Could you check a few things on this model? Use its own coordinates, in mm. Face numbers are marked on the shaded views. A direction names the side the tool comes from. Coordinates: 2 decimals unless noted, no trailing zeros. Write each loop counter-clockwise with the first axis right and the second up, starting at its lowest first coordinate (ties: lowest second). Pieces come first, ordered by that corner, then holes.
```python
from build123d import *

# Parameters (mm, degrees)
F1_DEPTH  = 41
F2_R      = 24.4692351537
F2_R_2    = 16.3
F3_DEPTH  = 25
F4_R      = 21.9531203574
F4_R_2    = 15
F5_DEPTH  = 9
F6_R      = 16.3
F7_DEPTH  = 7
F8_R      = 2.85
F9_DEPTH  = 41.001
F10_R     = 13.8
F11_DEPTH = 2.3
F12_R     = 6
F13_DEPTH = 41.001
F14_R     = 6.5
F15_DEPTH = 29
F16_R     = 2.5
F17_DEPTH = 13
F18_R     = 2.5
F19_DEPTH = 14.4
F21_D     = 4.2
F21_DEPTH = 8
F21_TIP   = 1.2618073
F22_R     = 3
F23_DEPTH = 29


with BuildPart() as f1:
    # F0 (on Front) → F1 (new body)
    with BuildSketch(Plane.XZ):
        Polygon((-18, -10.3923048454), (0, -20.7846096908), (18, -10.3923048454), (18, 10.3923048454), (0, 20.7846096908), (-18, 10.3923048454), align=None)
    extrude(amount=-F1_DEPTH)

    # F2 (on face) → F3 (cut)
    with BuildSketch(Plane(origin=(0, 41, 0), x_dir=(-1, 0, 0), z_dir=(0, 1, 0))):
        Circle(F2_R)
        Circle(F2_R_2, mode=Mode.SUBTRACT)
    extrude(amount=-F3_DEPTH, mode=Mode.SUBTRACT)

    # F4 (on face) → F5 (cut)
    with BuildSketch(Plane(origin=(0, 41, 0), x_dir=(-1, 0, 0), z_dir=(0, 1, 0))):
        Circle(F4_R)
        Circle(F4_R_2, mode=Mode.SUBTRACT)
    extrude(amount=-F5_DEPTH, mode=Mode.SUBTRACT)

    # F6 (on face) → F7 (join)
    with BuildSketch(Plane(origin=(0, 41, 0), x_dir=(-1, 0, 0), z_dir=(0, 1, 0))):
        Circle(F6_R)
    extrude(amount=-F7_DEPTH)

    # F8 (on face) → F9 (cut, through all)
    with BuildSketch(Plane.XZ):
        with Locations((8.5, 0)):
            Circle(F8_R)
        with Locations((4.87, -6.95)):
            Circle(F8_R)
    extrude(amount=-F9_DEPTH, mode=Mode.SUBTRACT)

    # F10 (on face) → F11 (cut)
    with BuildSketch(Plane(origin=(0, 41, 0), x_dir=(-1, 0, 0), z_dir=(0, 1, 0))):
        Circle(F10_R)
    extrude(amount=-F11_DEPTH, mode=Mode.SUBTRACT)

    # F12 (on face) → F13 (cut, through all)
    with BuildSketch(Plane.XZ):
        with Locations((-5, 0)):
            Circle(F12_R)
    extrude(amount=-F13_DEPTH, mode=Mode.SUBTRACT)

    # F14 (on face) → F15 (cut)
    with BuildSketch(Plane(origin=(0, 38.7, 0), x_dir=(-1, 0, 0), z_dir=(0, 1, 0))):
        with Locations((5, 0)):
            Circle(F14_R)
    extrude(amount=-F15_DEPTH, mode=Mode.SUBTRACT)

    # F16 (on face) → F17 (cut)
    with BuildSketch(Plane.XZ):
        with Locations((-0.1, 14.8379019182)):
            Circle(F16_R)
    extrude(amount=-F17_DEPTH, mode=Mode.SUBTRACT)

    # F18 (on face) → F19 (cut)
    with BuildSketch(Plane.XZ):
        with Locations((0.1, -14.8379019182)):
            Circle(F18_R)
    extrude(amount=-F19_DEPTH, mode=Mode.SUBTRACT)

    # F21
    with Locations(Plane(origin=(9, 0, 15.5884572681), x_dir=(0.8660254038, 0, -0.5), z_dir=(0.5, 0, 0.8660254038))):
        with Locations((4.4923048454, 5.9)):
            Hole(F21_D / 2, depth=F21_DEPTH)
            with Locations((0, 0, -(F21_DEPTH + F21_TIP / 2))):  # 118° drill point
                Cone(0, F21_D / 2, F21_TIP, mode=Mode.SUBTRACT)

    # F22 (on face) → F23 (cut)
    with BuildSketch(Plane(origin=(0, 38.7, 0), x_dir=(-1, 0, 0), z_dir=(0, 1, 0))):
        with Locations((-4.62, 7.15)):
            Circle(F22_R)
    extrude(amount=-F23_DEPTH, mode=Mode.SUBTRACT)


solid = f1.part
```
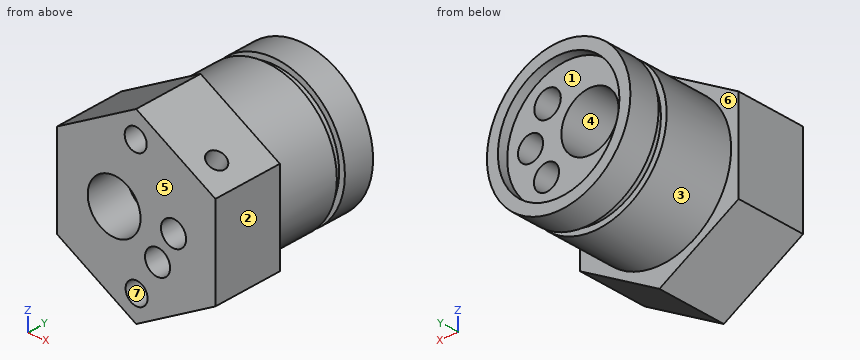
1. Please list where these lines run through material, in increasing order: line 1 along Z through (x, y) = (0, 6); line 2 along Y through (x, z) = (-16, -1.5); line 3 along Y through (x, z) = (0.5, 16).
Verdict:
line 1: z = -20.78 to -17.34, -12.34 to -3.32, 3.32 to 12.34, 17.34 to 20.78
line 2: y = 0 to 32, 34 to 41
line 3: y = 13 to 32, 34 to 41
2. For pin 1 (10 mm diameter, centred on x = -11.5, z = -4, fed in from +Y); pin 2 (17 mm diameter, centred on x = -5, z = 0, fed in from +Y); pin 3 (8 mm diameter, centred on x = -5, y = 22.5, fed in from +Z); pin 4 (8 mm diameter, centred on x = -7.5, y = 22, fed in from -Z), each with a flat end and sliding along its axis, tell me the tip position at first contact or that it passes through.
Verdict:
pin 1: stops at y = 41
pin 2: stops at y = 38.7
pin 3: stops at z = 16.27
pin 4: stops at z = -15.92
3. On a 3-axis mill with a long thin cutter (end or side, diameter ignored), from which of +Z, -Z, +X, -X, +Y, -Y can I reach the whole of each face in a straight line? I mean the marked faces 5, 6 and 7. Say none if no direction works.
Verdict:
face 5: +Z, -Z, +X, -X, -Y
face 6: +Y
face 7: -Y
4. I want a section at C-C on y = 28. Please give me the cut outline in (x, z).
Verdict:
outline: circle Ø32.6 at (0, 0); hole circle Ø13 at (-5, 0); hole circle Ø6 at (4.62, 7.15); hole circle Ø5.7 at (4.87, -6.95); hole circle Ø5.7 at (8.5, 0)
5. I want a section at B-B on x = 4.87. Please give me the cut outline in (y, z).
Verdict:
outline: (0, -17.97) - (16, -17.97) - (16, -15.56) - (32, -15.56) - (32, -14.19) - (34, -14.19) - (34, -15.56) - (41, -15.56) - (41, -12.91) - (38.7, -12.91) - (38.7, -9.8) - (0, -9.8) - close; (0, -4.1) - (38.7, -4.1) - (38.7, 4.16) - (9.7, 4.16) - (9.7, 10.14) - (38.7, 10.14) - (38.7, 12.91) - (41, 12.91) - (41, 15.56) - (34, 15.56) - (34, 14.19) - (32, 14.19) - (32, 15.56) - (16, 15.56) - (16, 17.97) - (0, 17.97) - close
6. I want a section at A-A on z = 0. Give the number of separate pieces and of enclosed holes in the cut face, plus the area to 3 significant figures.
Verdict:
separate pieces: 3
enclosed holes: 0
area: 608 mm2
7. If we mould it in two halves opening along X, with no side actions, what happens to the marked faces 1, 2, 3 and 4? For each: pulls with the +X half, pulls with the -X half, needs draft (parallel to the pull), parting line crosses it, or undercut.
Verdict:
face 1: undercut
face 2: pulls with the +X half
face 3: parting line crosses it
face 4: undercut
